Read the model definition and answer for the solid it produces. Units are mm, in the model's axes. A direction names the side the tool comes from. Coordinates: 2 decimals unless noted, no trailing zeros. Order: outer loops, then holes, each group sorted by start corner. A loop starts at its lowest first (then second) coordinate and runs counter-clockwise, first axis right, second up. Notation, with made-up numbers: (-14.5, 74.25) -> (23.5, 74.25) arc R34 ccw to (23.5, 104.25) -> close; hole circle Ø8 at (54.25, 31.5). An arc over 180 degrees is marked (long way). Use CSV: the item, a comma, the result in double quotes.
```python
from build123d import *

# Parameters (mm, degrees)
BOSS_EXTRUDE1_DEPTH = 15.24
SKETCH5_R           = 1.143
SKETCH5_R_2         = 2.54
CUT_EXTRUDE1_DEPTH  = 15.24
SKETCH6_R           = 1.778
CUT_EXTRUDE2_DEPTH  = 15.24


with BuildPart() as part:
    # Sketch2 → Boss-Extrude1 (new body)
    with BuildSketch(Plane.XY):
        Polygon((-27.94, 0), (27.94, 0), (27.94, 6.35), (-2.54, 6.35), (-2.54, 50.8), (-8.89, 50.8), (-8.89, 6.35), (-27.94, 6.35), align=None)
    extrude(amount=BOSS_EXTRUDE1_DEPTH)

    # Sketch5 → Cut-Extrude1 (cut)
    with BuildSketch(Plane.ZY.offset(8.89)):
        with Locations((7.62, 32.766)):
            Circle(SKETCH5_R)
        with Locations((7.62, 27.686)):
            Circle(SKETCH5_R_2)
        with Locations((12.7, 27.686)):
            Circle(SKETCH5_R)
        with Locations((7.62, 22.606)):
            Circle(SKETCH5_R)
        with Locations((2.54, 27.686)):
            Circle(SKETCH5_R)
    extrude(amount=-CUT_EXTRUDE1_DEPTH, mode=Mode.SUBTRACT)

    # Sketch6 → Cut-Extrude2 (cut)
    with BuildSketch(Plane(origin=(0, 6.35, 0), x_dir=(1, 0, 0), z_dir=(0, 1, 0))):
        with Locations((-25.146, -7.62)):
            Circle(SKETCH6_R)
        with Locations((-15.24, -7.62)):
            Circle(SKETCH6_R)
    extrude(amount=-CUT_EXTRUDE2_DEPTH, mode=Mode.SUBTRACT)


solid = part.part
```
Item 1: Find section A-A, the plane z = 12.7. Give the vertices of the cut face in (x, y), then the cut area to 3 significant figures.
Return value:
outline,"(-27.94, 0) -> (27.94, 0) -> (27.94, 6.35) -> (-2.54, 6.35) -> (-2.54, 26.54) -> (-8.89, 26.54) -> (-8.89, 6.35) -> (-27.94, 6.35) -> close; (-8.89, 28.83) -> (-2.54, 28.83) -> (-2.54, 50.8) -> (-8.89, 50.8) -> close"
area,"623 mm^2"
Item 2: Straight lines are drawn through the part: line 1 along Y through (x, z) = (-5, 7.62); line 2 along X through (y, z) = (3.5, 7.62); line 3 along Y through (x, z) = (-4, 12.7). For each, find the intervals that lie inside material, in ascending order.
Return value:
line 1,"y = 0 to 21.46, 23.75 to 25.15, 30.23 to 31.62, 33.91 to 50.8"
line 2,"x = -27.94 to -26.92, -23.37 to -17.02, -13.46 to 27.94"
line 3,"y = 0 to 26.54, 28.83 to 50.8"
Item 3: Find section D-D, the plane y = 24.5. Give the vertices of the cut face in (x, z), then the cut area to 3 significant figures.
Return value:
outline,"(-8.89, 0) -> (-2.54, 0) -> (-2.54, 15.24) -> (-8.89, 15.24) -> close"
area,"96.8 mm^2"
Item 4: The mould has two halves that part along Y. Classify faces 4 (the cylindrical face through (-26.922, 3.219, 7.542)), 5 (the flat face through (13, 6.35, 8)), 6 (the cylindrical face through (-5.76, 23.74, 7.47)): +Y half, -Y half, draft (parallel to the pull), parting line (faces both ways), or undercut.
Return value:
face 4,"draft"
face 5,"+Y half"
face 6,"undercut"
Item 5: Each of these flat-tipped pins is pushed along its axis until it touches: P1, Ø4.5, axis at x = -15.24, z = 7.62, coming from the +Y side; P2, Ø8, axis at y = 27.686, z = 7.62, coming from the -X side; P3, Ø2, axis at y = 17.5, z = 5, coming from the +X side; P4, Ø2, axis at y = 22.606, z = 7.62, coming from the +X side. Where does it stop, or does it pass through?
Return value:
P1,"stops at y = 6.35"
P2,"stops at x = -8.89"
P3,"stops at x = -2.54"
P4,"passes through"
Item 6: Find section B-B, the plane x = -15.24. Give the vertices of the cut face in (y, z).
Return value:
outline,"(0, 0) -> (6.35, 0) -> (6.35, 5.84) -> (0, 5.84) -> close; (0, 9.4) -> (6.35, 9.4) -> (6.35, 15.24) -> (0, 15.24) -> close"
Item 7: Find section C-C, the plane z = 7.62. Give the vertices of the cut face in (x, y), then the cut area to 3 significant figures.
Return value:
outline,"(-27.94, 0) -> (-26.92, 0) -> (-26.92, 6.35) -> (-27.94, 6.35) -> close; (-23.37, 0) -> (-17.02, 0) -> (-17.02, 6.35) -> (-23.37, 6.35) -> close; (-13.46, 0) -> (27.94, 0) -> (27.94, 6.35) -> (-2.54, 6.35) -> (-2.54, 21.46) -> (-8.89, 21.46) -> (-8.89, 6.35) -> (-13.46, 6.35) -> close; (-8.89, 23.75) -> (-2.54, 23.75) -> (-2.54, 25.15) -> (-8.89, 25.15) -> close; (-8.89, 30.23) -> (-2.54, 30.23) -> (-2.54, 31.62) -> (-8.89, 31.62) -> close; (-8.89, 33.91) -> (-2.54, 33.91) -> (-2.54, 50.8) -> (-8.89, 50.8) -> close"
area,"531 mm^2"
Item 8: A tool of negligible diameter and unlimited length cuts with its end or side. For faces 1 (the flat face through (-18, 6.35, 8)), 2 (the cylindrical face through (-5.76, 28.82, 2.39)), 3 (the flat face through (-2.54, 28, 11)), from which of +Z, -Z, +X, -X, +Y, -Y can it reach the whole face along a straight path? Write none if from no direction.
Return value:
face 1,"+Z, -Z, -X, +Y"
face 2,"+X, -X"
face 3,"+Z, -Z, +X, +Y"
